Build history of the part. All positions in model axes, mm. Coordinates: 2 decimals unless noted, no trailing zeros. Write each loop counter-clockwise with the first axis right and the second up, starting at its lowest first coordinate (ties: lowest second). Pieces come first, ordered by that corner, then holes.
```python
from build123d import *

# Parameters (mm, degrees)
F0_W     = 4.1
F0_H     = 2.55
F0_W_2   = 3.1
F0_H_2   = 1.55
F3_DEPTH = 300
F4_R     = 9.525
F4_W     = 4.1
F4_H     = 2.55
F5_DEPTH = 6.35
F6_R     = 9.525
F6_W     = 4.1
F6_H     = 2.55
F7_DEPTH = 6.35


with BuildPart() as f3:
    # F0 (on Front) → F3 (new body)
    with BuildSketch(Plane.XZ):
        Rectangle(F0_W, F0_H)
        Rectangle(F0_W_2, F0_H_2, mode=Mode.SUBTRACT)
    extrude(amount=F3_DEPTH)

    # F4 (on face) → F5 (join)
    with BuildSketch(Plane.XZ.offset(300)):
        Circle(F4_R)
        Rectangle(F4_W, F4_H, mode=Mode.SUBTRACT)
    extrude(amount=-F5_DEPTH)

    # F6 (on face) → F7 (join)
    with BuildSketch(Plane.XZ):
        Circle(F6_R)
        Rectangle(F6_W, F6_H, mode=Mode.SUBTRACT)
    extrude(amount=F7_DEPTH)


solid = f3.part
```
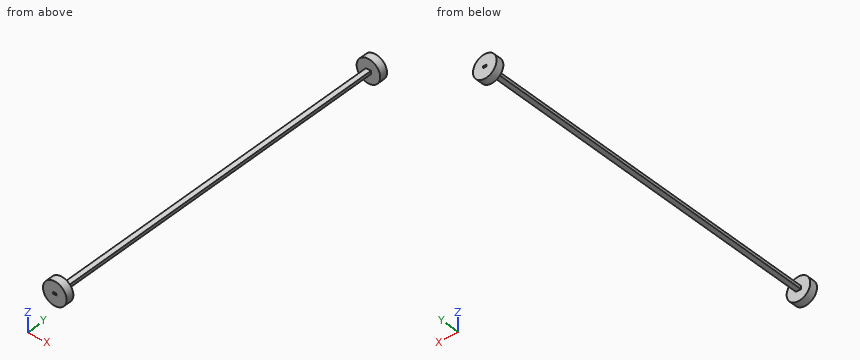
1. Saw through at A-A on y = -57.5. List the corners of the cut face in (x, z) (3 decimals), plus the area to 3 significant figures.
Computed values:
outline: (-2.05, -1.275) - (2.05, -1.275) - (2.05, 1.275) - (-2.05, 1.275) - close; hole (-1.55, -0.775) - (1.55, -0.775) - (1.55, 0.775) - (-1.55, 0.775) - close
area: 5.65 mm2
2. Probe line 1 along Z through (x, y) = (0.5, -173.5) (3 decimals); line 2 along Y through (x, z) = (-5.5, -2). List the from-to ranges inside material, lowest first.
Computed values:
line 1: z = -1.275 to -0.775, 0.775 to 1.275
line 2: y = -300 to -293.65, -6.35 to 0
3. Flat gauge pins, fed straight in: pin 1 (1.5 mm diameter, centred on x = 4, y = -45, fed in from -Z); pin 2 (1.6 mm diameter, centred on x = 0.5, y = -115.5, fed in from +Z) (3 decimals); pin 3 (10 mm diameter, centred on y = -216, z = -2, fed in from +X); pin 4 (0.8 mm diameter, centred on y = -128.5, z = 0, fed in from -X). Where does each tip first touch, or does it go through?
Computed values:
pin 1: passes through
pin 2: stops at z = 1.275
pin 3: stops at x = 2.05
pin 4: stops at x = -2.05
4. Saw through at C-C on x = 4.75. List the corners of the cut face in (y, z).
Computed values:
outline: (-300, -8.26) - (-293.65, -8.26) - (-293.65, 8.26) - (-300, 8.26) - close; (-6.35, -8.26) - (0, -8.26) - (0, 8.26) - (-6.35, 8.26) - close
5. Saw through at B-B on z = 6.5. List the corners of the cut face in (x, y), plus the area to 3 significant figures.
Computed values:
outline: (-6.96, -300) - (6.96, -300) - (6.96, -293.65) - (-6.96, -293.65) - close; (-6.96, -6.35) - (6.96, -6.35) - (6.96, 0) - (-6.96, 0) - close
area: 177 mm2
